Verification items for the finished model (mm, model axes). Face numbers are marked on the shaded views. A direction names the side the tool comes from. Coordinates: 2 decimals unless noted, no trailing zeros. Order: outer loops, then holes, each group sorted by start corner. A loop starts at its lowest first (then second) coordinate and runs counter-clockwise, first axis right, second up. Notation, with made-up numbers: (-30, -34.5) -> (-1, -34.5) arc R15 ccw to (-1, -19.5) -> close; hole circle Ø6 at (48.5, 68). An arc over 180 degrees is marked (long way). Write item = value, one per line. Start each with the question number.
1. Go/stop test with flat-tipped pins: P1, Ø2, axis at y = -22.5, z = 13.5, coming from the +X side; P2, Ø1.5, axis at y = -7.5, z = -13.5, coming from the +X side; P3, Ø1, axis at y = -17, z = -16, coming from the +X side. Record where each tip stops, or that it passes through.
2. Set-up check for the marked faces 1, 2, 3 and 4: record each of +Z, -Z, +X, -X, +Y, -Y from which the full face is reachable in a straight line by a thin tool's end or side.
3. Cross-section at B-B on z = 11. Record the cut outline in (x, y), plus the area to 3 significant figures.
4. Cross-section at C-C on z = -15. Record the cut outline in (x, y).
5. Thickness scan on line 1 along Z through (x, y) = (-9, -19); line 2 along X through (y, z) = (-1, 12); line 3 along Y through (x, z) = (-9.5, -27). Record the ranges inside material, lowest first. Write a range as from..to.
6. Release check for a two-part mould opening along X. For the marked faces 5, 6, 7 and 8 record: +X half, -X half, draft (parallel to the pull), parting line (faces both ways), or undercut.
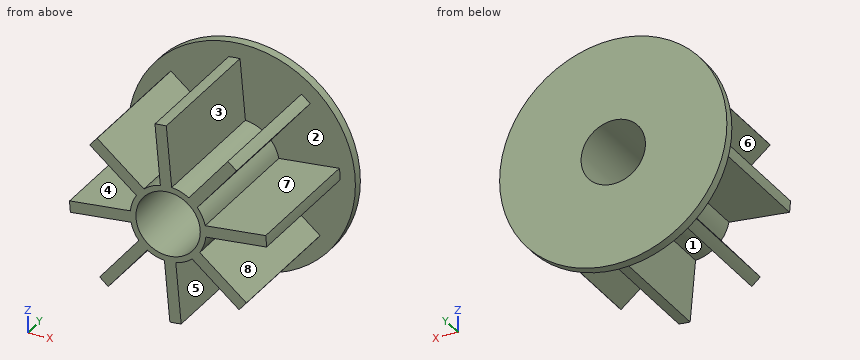
from build123d import *

# Parameters (mm, degrees)
F0_R     = 30
F0_R_2   = 8.5
F1_DEPTH = 2.5
F3_DEPTH = 37
F4_DEPTH = 40


with BuildPart() as f1:
    # F0 (on Front) → F1 (new body)
    with BuildSketch(Plane.XZ):
        Circle(F0_R)
        Circle(F0_R_2, mode=Mode.SUBTRACT)
    extrude(amount=-F1_DEPTH)

    # F2 (on Front) → F3 (join)
    with BuildSketch(Plane.XZ):
        with BuildLine():
            ThreePointArc((9.9539621754, -0.9584555339), (9.9884839128, -0.4797802861), (10, 0))
            ThreePointArc((10, 0), (9.9474412154, 1.0239205366), (9.790317347, 2.0370778693))
            ThreePointArc((9.790317347, 2.0370778693), (9.0162927853, 4.3250970404), (7.7162445614, 6.3607837464))
            ThreePointArc((7.7162445614, 6.3607837464), (6.6748253827, 7.4462545021), (5.4823682108, 8.3632313612))
            ThreePointArc((5.4823682108, 8.3632313612), (3.3171763231, 9.4337872163), (0.9584555339, 9.9539621754))
            ThreePointArc((0.9584555339, 9.9539621754), (-0.5454827615, 9.9851113442), (-2.0370778693, 9.790317347))
            ThreePointArc((-2.0370778693, 9.790317347), (-4.3250970404, 9.0162927853), (-6.3607837464, 7.7162445614))
            ThreePointArc((-6.3607837464, 7.7162445614), (-7.4462545021, 6.6748253827), (-8.3632313612, 5.4823682108))
            ThreePointArc((-8.3632313612, 5.4823682108), (-9.4337872163, 3.3171763231), (-9.9539621754, 0.9584555339))
            ThreePointArc((-9.9539621754, 0.9584555339), (-9.9851113442, -0.5454827615), (-9.790317347, -2.0370778693))
            ThreePointArc((-9.790317347, -2.0370778693), (-9.0162927853, -4.3250970404), (-7.7162445614, -6.3607837464))
            ThreePointArc((-7.7162445614, -6.3607837464), (-6.6748253827, -7.4462545021), (-5.4823682108, -8.3632313612))
            ThreePointArc((-5.4823682108, -8.3632313612), (-3.3171763231, -9.4337872163), (-0.9584555339, -9.9539621754))
            ThreePointArc((-0.9584555339, -9.9539621754), (0.5454827615, -9.9851113442), (2.0370778693, -9.790317347))
            ThreePointArc((2.0370778693, -9.790317347), (4.3250970404, -9.0162927853), (6.3607837464, -7.7162445614))
            ThreePointArc((6.3607837464, -7.7162445614), (7.4462545021, -6.6748253827), (8.3632313612, -5.4823682108))
            ThreePointArc((8.3632313612, -5.4823682108), (9.4337872163, -3.3171763231), (9.9539621754, -0.9584555339))
        make_face()
        with BuildLine():
            ThreePointArc((-8.3632313612, 5.4823682108), (-7.4462545021, 6.6748253827), (-6.3607837464, 7.7162445614))
            Line((-6.3607837464, 7.7162445614), (-18.7140811189, 18.0494644761))
            ThreePointArc((-18.7140811189, 18.0494644761), (-19.7242264231, 16.9397429736), (-20.6686668466, 15.7735921965))
            Line((-20.6686668466, 15.7735921965), (-8.3632313612, 5.4823682108))
        make_face()
        with BuildLine():
            Line((-15.7735921965, -20.6686668466), (-5.4823682108, -8.3632313612))
            ThreePointArc((-5.4823682108, -8.3632313612), (-6.6748253827, -7.4462545021), (-7.7162445614, -6.3607837464))
            Line((-7.7162445614, -6.3607837464), (-18.0494644761, -18.7140811189))
            ThreePointArc((-18.0494644761, -18.7140811189), (-16.9397429736, -19.7242264231), (-15.7735921965, -20.6686668466))
        make_face()
        with BuildLine():
            Line((3.4613404795, -25.7685684912), (2.0370778693, -9.790317347))
            ThreePointArc((2.0370778693, -9.790317347), (0.5454827615, -9.9851113442), (-0.9584555339, -9.9539621754))
            Line((-0.9584555339, -9.9539621754), (0.469954935, -25.9957523907))
            ThreePointArc((0.469954935, -25.9957523907), (1.9689271292, -25.9253413856), (3.4613404795, -25.7685684912))
        make_face()
        with BuildLine():
            Line((20.6686668466, -15.7735921965), (8.3632313612, -5.4823682108))
            ThreePointArc((8.3632313612, -5.4823682108), (7.4462545021, -6.6748253827), (6.3607837464, -7.7162445614))
            Line((6.3607837464, -7.7162445614), (18.7140811189, -18.0494644761))
            ThreePointArc((18.7140811189, -18.0494644761), (19.7242264231, -16.9397429736), (20.6686668466, -15.7735921965))
        make_face()
        with BuildLine():
            ThreePointArc((9.790317347, 2.0370778693), (9.9474412154, 1.0239205366), (10, 0))
            ThreePointArc((10, 0), (9.9884839128, -0.4797802861), (9.9539621754, -0.9584555339))
            Line((9.9539621754, -0.9584555339), (25.9957523907, 0.469954935))
            ThreePointArc((25.9957523907, 0.469954935), (25.9253413856, 1.9689271292), (25.7685684912, 3.4613404795))
            Line((25.7685684912, 3.4613404795), (9.790317347, 2.0370778693))
        make_face()
        with BuildLine():
            ThreePointArc((5.4823682108, 8.3632313612), (6.6748253827, 7.4462545021), (7.7162445614, 6.3607837464))
            Line((7.7162445614, 6.3607837464), (18.0494644761, 18.7140811189))
            ThreePointArc((18.0494644761, 18.7140811189), (16.9397429736, 19.7242264231), (15.7735921965, 20.6686668466))
            Line((15.7735921965, 20.6686668466), (5.4823682108, 8.3632313612))
        make_face()
        with BuildLine():
            ThreePointArc((-2.0370778693, 9.790317347), (-0.5454827615, 9.9851113442), (0.9584555339, 9.9539621754))
            Line((0.9584555339, 9.9539621754), (-0.469954935, 25.9957523907))
            ThreePointArc((-0.469954935, 25.9957523907), (-1.9689271292, 25.9253413856), (-3.4613404795, 25.7685684912))
            Line((-3.4613404795, 25.7685684912), (-2.0370778693, 9.790317347))
        make_face()
        with BuildLine():
            ThreePointArc((-9.790317347, -2.0370778693), (-9.9851113442, -0.5454827615), (-9.9539621754, 0.9584555339))
            Line((-9.9539621754, 0.9584555339), (-25.9957523907, -0.469954935))
            ThreePointArc((-25.9957523907, -0.469954935), (-25.9253413856, -1.9689271292), (-25.7685684912, -3.4613404795))
            Line((-25.7685684912, -3.4613404795), (-9.790317347, -2.0370778693))
        make_face()
    extrude(amount=F3_DEPTH)

    # F4 (cut): a face of the model
    f4_faces = [f1.faces().sort_by_distance(p)[0] for p in [
        (0, 0, 0),
    ]]
    extrude(f4_faces, amount=-F4_DEPTH, mode=Mode.SUBTRACT)


solid = f1.part
Worked out:
q1.P1 = 14.52
q1.P2 = 18.85
q1.P3 = 20.67
q2.face_1 = -Z, -Y
q2.face_2 = -Y
q2.face_3 = +Z, -Y
q2.face_4 = -X, -Y
q3.outline = (-27.91, 0) -> (-14.96, 0) -> (-14.96, -37) -> (-10.29, -37) -> (-10.29, 0) -> (-2.14, 0) -> (-2.14, -37) -> (0.87, -37) -> (0.87, 0) -> (7.69, 0) -> (7.69, -37) -> (11.6, -37) -> (11.6, 0) -> (27.91, 0) -> (27.91, 2.5) -> (-27.91, 2.5) -> close
q3.area = 569 mm²
q4.outline = (-25.98, 0) -> (-14.94, 0) -> (-14.94, -37) -> (-11.03, -37) -> (-11.03, 0) -> (-0.51, 0) -> (-0.51, -37) -> (2.5, -37) -> (2.5, 0) -> (15.07, 0) -> (15.07, -37) -> (19.74, -37) -> (19.74, 0) -> (25.98, 0) -> (25.98, 2.5) -> (-25.98, 2.5) -> close
q5.line_1 = -12.57..-7.9, -4.36..4.36, 6.01..9.92
q5.line_2 = -16.16..-11.48, -2.23..0.78, 8.52..12.43
q5.line_3 = 0..2.5
q6.face_5 = undercut
q6.face_6 = -X half
q6.face_7 = undercut
q6.face_8 = +X half
